Part print with two shaded views. Sizes in mm from the minimum x, y, z corner. Round coordinates to 2 decimals unless told otherwise and drop trailing zeros. Order: outer loops, then holes, each group sorted by start corner. A loop starts at its lowest first (then second) coordinate and runs counter-clockwise, first axis right, second up. Notation, with made-up numbers: M -11.5,-13 L -4.5,-13 A19 ccw -4.5,4 Z; hole C 88.25,46 d8. An arc over 180 degrees is marked long. Return JSON: item names as keys, results as strings. Group by question number.
Item 1: Slice it at C-C on z = 2.35. Write the cut outline in (x, y).
Item 2: Probe line 1 along X through (y, z) = (40.5, 1.55); line 2 along Y through (x, z) = (38.5, 1.85); line 3 along X through (y, z) = (3.5, 2.25). List the from-to ranges inside material, lowest first.
Item 3: Slice it at A-A on x = 38.5. Write the cut outline in (y, z), then the cut area to 3 significant figures.
Item 4: Pin check, flat tips, straight feed: pin 1 Ø2 at (x, y) = (38.5, 40.5) entering from +Z; pin 2 Ø1.4 at (x, y) = (38.5, 3.5) entering from +Z; pin 3 Ø1 at (x, y) = (21.5, 26.5) entering from -Z; pin 4 Ø1.5 at (y, z) = (26.5, 1) entering from -X. Stop position of each tip, or through.
Item 5: Slice it at D-D on x = 32. Write the cut outline in (y, z), then the cut area to 3 significant figures.
Item 6: Slice it at B-B on y = 3.5. Write the cut outline in (x, z).
Item 7: Pull direction Y, two halves, no side cores. Call the marked faces 1 and 2: pulls with the +Y half, pulls with the -Y half, needs draft (parallel to the pull), parting line crosses it, or undercut.
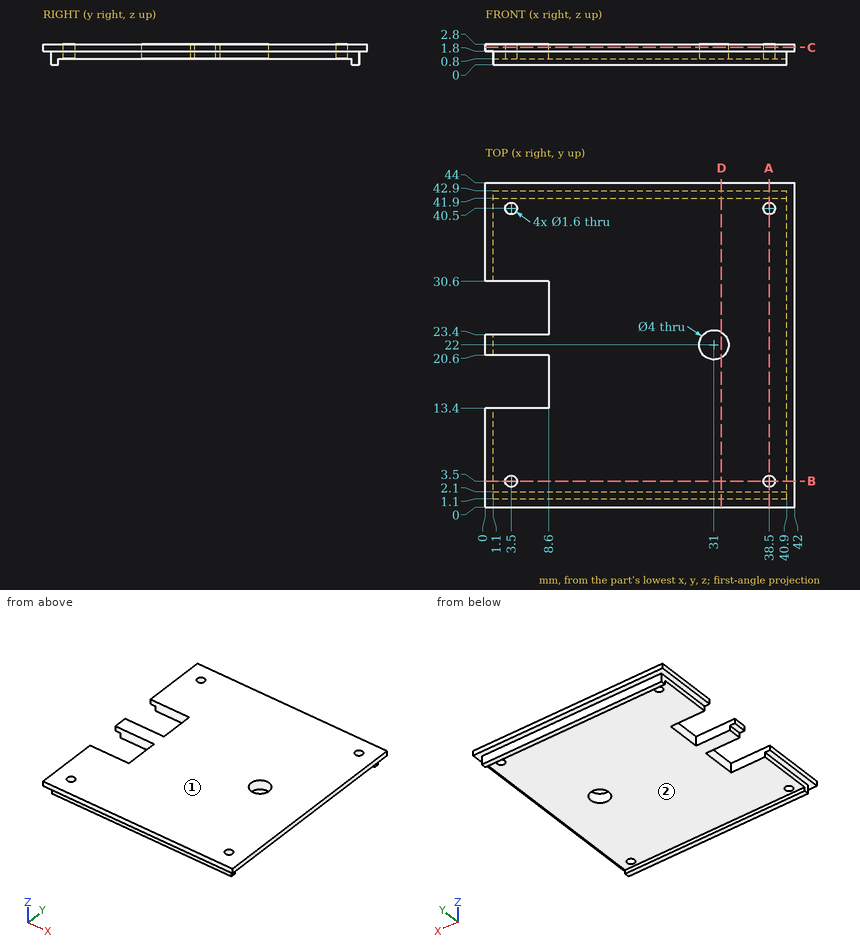
Output values:
{
 "1": {"outline": "M 0,0 L 42,0 L 42,44 L 0,44 L 0,30.6 L 8.6,30.6 L 8.6,23.4 L 0,23.4 L 0,20.6 L 8.6,20.6 L 8.6,13.4 L 0,13.4 Z; hole C 3.5,3.5 d1.6; hole C 3.5,40.5 d1.6; hole C 31,22 d4; hole C 38.5,3.5 d1.6; hole C 38.5,40.5 d1.6"},
 "2": {"line 1": "1.1 to 2.7, 4.3 to 37.7, 39.3 to 40.9", "line 2": "0 to 2.7, 4.3 to 39.7, 41.3 to 44", "line 3": "0 to 2.7, 4.3 to 37.7, 39.3 to 42"},
 "3": {"outline": "M 0,1.8 L 1.1,1.8 L 1.1,0 L 2.1,0 L 2.1,0.8 L 2.7,0.8 L 2.7,2.8 L 0,2.8 Z; M 4.3,0.8 L 39.7,0.8 L 39.7,2.8 L 4.3,2.8 Z; M 41.3,0.8 L 41.9,0.8 L 41.9,0 L 42.9,0 L 42.9,1.8 L 44,1.8 L 44,2.8 L 41.3,2.8 Z", "area": "81.0 mm²"},
 "4": {"pin 1": "z = 2.8", "pin 2": "through", "pin 3": "z = 0.8", "pin 4": "x = 8.6"},
 "5": {"outline": "M 0,1.8 L 1.1,1.8 L 1.1,0 L 2.1,0 L 2.1,0.8 L 20.27,0.8 L 20.27,2.8 L 0,2.8 Z; M 23.73,0.8 L 41.9,0.8 L 41.9,0 L 42.9,0 L 42.9,1.8 L 44,1.8 L 44,2.8 L 23.73,2.8 Z", "area": "80.5 mm²"},
 "6": {"outline": "M 0,1.8 L 1.1,1.8 L 1.1,0.8 L 2.7,0.8 L 2.7,2.8 L 0,2.8 Z; M 4.3,0.8 L 37.7,0.8 L 37.7,2.8 L 4.3,2.8 Z; M 39.3,0.8 L 40.9,0.8 L 40.9,1.8 L 42,1.8 L 42,2.8 L 39.3,2.8 Z"},
 "7": {"face 1": "needs draft", "face 2": "undercut"}
}
